from build123d import *

# Parameters (mm, degrees)
SKETCH1_R           = 2.5
SKETCH1_R_2         = 1.25
BOSS_EXTRUDE1_DEPTH = 5
SKETCH2_R           = 1.25
CUT_EXTRUDE1_DEPTH  = 10.354143467


with BuildPart() as part:
    # Sketch1 → Boss-Extrude1 (new body)
    # profile 1 of 2: a face of its own
    with BuildSketch(Plane.XY):
        with BuildLine():
            ThreePointArc((2.5, 0), (0, -2.5), (-2.5, 0))
            Line((-2.5, 0), (-2.5, -5))
            Line((-2.5, -5), (2.5, -5))
            Line((2.5, -5), (2.5, 0))
        make_face()
    # profile 2 of 2: a face of its own
    with BuildSketch(Plane.XY):
        Circle(SKETCH1_R)
        Circle(SKETCH1_R_2, mode=Mode.SUBTRACT)
    extrude(amount=BOSS_EXTRUDE1_DEPTH)

    # Sketch2 → Cut-Extrude1 (cut, through all)
    with BuildSketch(Plane.XZ.offset(5)):
        with Locations(Location((0, 2.5, 0), (0, 0, 270))):
            Circle(SKETCH2_R)
    extrude(amount=-CUT_EXTRUDE1_DEPTH, mode=Mode.SUBTRACT)


solid = part.part
Source: CAD feature listing. Evaluate the final solid. Frame: model axes, mm. Coordinates: 2 decimals unless noted, no trailing zeros. Order: outer loops, then holes, each group sorted by start corner. A loop starts at its lowest first (then second) coordinate and runs counter-clockwise, first axis right, second up.
Item 1: Pull-direction query (X, two-part tool) for faces 1 (the face through (2.5, -3, 2)), 2 (the face through (0.38, -3.09, 1.31)), 3 (the face through (0, -2, 0)); classes: pulls with the +X half, pulls with the -X half, needs draft (parallel to the pull), parting line crosses it, or undercut.
Output values:
face 1: pulls with the +X half
face 2: undercut
face 3: needs draft
Item 2: Cut plane C-C (z = 4.5). Return loops of the section in (x, y).
Output values:
outline: (-2.5, -5) - (2.5, -5) - (2.5, 0) arc R2.5 ccw to (-2.5, 0) - close; hole circle Ø2.5 at (0, 0)
Item 3: Cut plane A-A (x = 0). Return loops of the section in (y, z), plus the area to 3 significant figures.
Output values:
outline: (-5, 0) - (-1.25, 0) - (-1.25, 1.25) - (-5, 1.25) - close; (-5, 3.75) - (-1.25, 3.75) - (-1.25, 5) - (-5, 5) - close; (1.25, 0) - (2.5, 0) - (2.5, 1.25) - (1.25, 1.25) - close; (1.25, 3.75) - (2.5, 3.75) - (2.5, 5) - (1.25, 5) - close
area: 12.5 mm2
Item 4: First-contact query: P1, Ø1.5, axis at x = 0, z = 2.5, coming from the -Y side; P2, Ø3, axis at x = 2, z = 2.5, coming from the +Y side. Flat tips, straight axial feed; report the tip coordinate or a pass-through.
Output values:
P1: passes through
P2: stops at y = 2.36
Item 5: Material intervals for line 1 (X direction, y = -0.5, z = 2.5); line 2 (Z direction, x = 0, y = -2.05); line 3 (Y direction, x = 0.3, z = 3.95), sorted ascending.
Output values:
line 1: x = -2.5 to -1.25, 1.25 to 2.5
line 2: z = 0 to 1.25, 3.75 to 5
line 3: y = -5 to -1.21, 1.21 to 2.48
Item 6: Cut plane B-B (y = 1.5). Return loops of the section in (x, z), plus the area to 3 significant figures.
Output values:
outline: (-2, 0) - (2, 0) - (2, 5) - (-2, 5) - close; hole circle Ø2.5 at (0, 2.5)
area: 15.1 mm2
Item 7: Cut plane D-D (x = 1.1). Return loops of the section in (y, z) (3 decimals), plus the area to 3 significant figures.
Output values:
outline: (-5, 0) - (-0.594, 0) - (-0.594, 1.906) - (-5, 1.906) - close; (-5, 3.094) - (-0.594, 3.094) - (-0.594, 5) - (-5, 5) - close; (0.594, 0) - (2.245, 0) - (2.245, 1.906) - (0.594, 1.906) - close; (0.594, 3.094) - (2.245, 3.094) - (2.245, 5) - (0.594, 5) - close
area: 23.1 mm2
